Here's how the part is built. I have some questions about the finished solid (model axes, mm). Face numbers are marked on the shaded views. Round coordinates to 2 decimals unless told otherwise and drop trailing zeros. Write each question's results on one line, items separated by ' | '. Start each with the question number.
```python
from build123d import *

# Parameters (mm, degrees)
PAD_DEPTH   = 22
FILLET_R    = 21
FILLET001_R = 21
FILLET002_R = 21
FILLET003_R = 21


with BuildPart() as part:
    # Sketch → Pad (new body)
    with BuildSketch(Plane.XY):
        with BuildLine():
            Line((940, 362), (940, 0))
            Line((940, 0), (0, 0))
            Line((0, 0), (0, 362))
            ThreePointArc((940, 362), (470, 380), (0, 362))
        make_face()
    extrude(amount=PAD_DEPTH)

    # Fillet
    fillet_edges = [part.edges().sort_by_distance(p)[0] for p in [
        (470, 380, 22),
    ]]
    fillet(fillet_edges, radius=FILLET_R)

    # Fillet001
    fillet001_edges = [part.edges().sort_by_distance(p)[0] for p in [
        (470, 0, 22),
    ]]
    fillet(fillet001_edges, radius=FILLET001_R)

    # Fillet002
    fillet002_edges = [part.edges().sort_by_distance(p)[0] for p in [
        (0, 180.969047, 22),
    ]]
    fillet(fillet002_edges, radius=FILLET002_R)

    # Fillet003
    fillet003_edges = [part.edges().sort_by_distance(p)[0] for p in [
        (940, 180.969047, 22),
    ]]
    fillet(fillet003_edges, radius=FILLET003_R)


solid = part.part
```
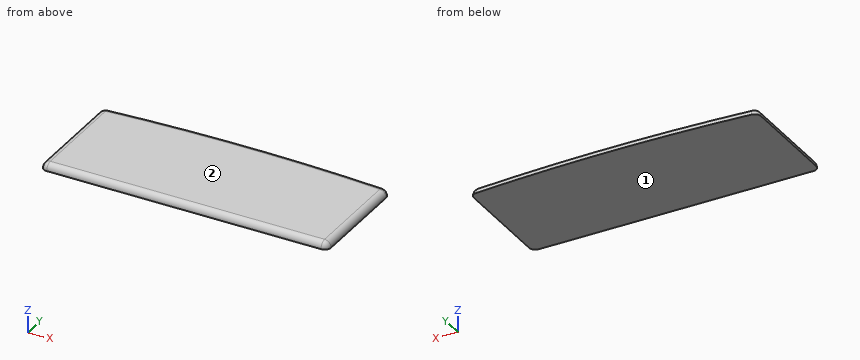
Item 1: I need wall thicknesses on L1, parallel to Y at x = 438.5, z = 2.5; L2, parallel to X at y = 200, z = 15.25; L3, parallel to Y at x = 83, z = 14. Which ranges of each line are inside material? Lowest first, please.
Item 2: If we mould it in two halves opening along Z, with no side actions, what happens to the marked faces 1 and 2? For each: released by +Z, released by -Z, zero draft, split by the parting line, or undercut.
Item 3: I'm going to push flat-ended pins straight in: pin 1 (10 mm diameter, centred on y = 226.5, z = 6.5, fed in from +X); pin 2 (4 mm diameter, centred on y = 330.5, z = 17.5, fed in from -X); pin 3 (4 mm diameter, centred on y = 216, z = 6.5, fed in from +X). Where does each tip first touch, or does it pass through?
Numbers:
1) L1: 0.05 to 379.87 | L2: 5.57 to 934.43 | L3: 4.51 to 363.29
2) face 1: released by -Z | face 2: released by +Z
3) pin 1: x = 939.99 | pin 2: x = 5.81 | pin 3: x = 939.71
